Source: CAD feature listing. Evaluate the final solid. Frame: model axes, mm. Face numbers are marked on the shaded views. Give positions to 0.01 mm unless a question says otherwise; leave off trailing zeros. Write each loop counter-clockwise with the first axis right and the second up, starting at its lowest first coordinate (ties: lowest second). Pieces come first, ordered by that corner, then holes. Notation, with made-up numbers: M 41.5,-37 L 94.5,-37 A30 cw 94.5,-9 Z; hole C 30,-15.5 d5. An arc over 180 degrees is marked long. Return JSON: item names as keys, results as strings.
```python
from build123d import *

# Parameters (mm, degrees)
F0_W     = 88.9
F0_H     = 101.6
F1_DEPTH = 6.35
F2_R     = 5.08
F3_T     = -2.54
F4_W     = 83.82
F4_H     = 2.54
F5_DEPTH = 10.16
F7_DEPTH = 6.35
F8_R     = 5.08


with BuildPart() as f1:
    # F0 (on Front) → F1 (new body, symmetric)
    with BuildSketch(Plane.XZ):
        with Locations((0, 50.8)):
            Rectangle(F0_W, F0_H)
    extrude(amount=F1_DEPTH, both=True)

    # F2
    f2_edges = [f1.edges().sort_by_distance(p)[0] for p in [
        (-44.45, 0, 0),
        (44.45, 0, 0),
    ]]
    fillet(f2_edges, radius=F2_R)

    # F3
    f3_openings = [f1.faces().sort_by_distance(p)[0] for p in [
        (0, -6.35, 50.860979),
    ]]
    offset(amount=F3_T, openings=f3_openings)

    # F4 (on face) → F5 (cut, through all)
    with BuildSketch(Plane.XZ.offset(6.35)):
        with Locations((0, 100.33)):
            Rectangle(F4_W, F4_H)
    extrude(amount=-F5_DEPTH, mode=Mode.SUBTRACT)

    # F6 (on face) → F7 (join)
    with BuildSketch(Plane.XZ.offset(-3.81)):
        with BuildLine():
            Line((38.735, 5.715), (-38.735, 5.715))
            Line((-38.735, 5.715), (-38.735, 101.6))
            Line((-38.735, 101.6), (-41.91, 101.6))
            Line((-41.91, 101.6), (-41.91, 5.08))
            ThreePointArc((-41.91, 5.08), (-41.1660512242, 3.2839487758), (-39.37, 2.54))
            Line((-39.37, 2.54), (39.37, 2.54))
            ThreePointArc((39.37, 2.54), (41.1660512242, 3.2839487758), (41.91, 5.08))
            Line((41.91, 5.08), (41.91, 101.6))
            Line((41.91, 101.6), (38.735, 101.6))
            Line((38.735, 101.6), (38.735, 5.715))
        make_face()
    extrude(amount=F7_DEPTH)

    # F8
    f8_edges = [f1.edges().sort_by_distance(p)[0] for p in [
        (-38.735, 0.635, 5.715),
        (38.735, 0.635, 5.715),
    ]]
    fillet(f8_edges, radius=F8_R)


solid = f1.part
```
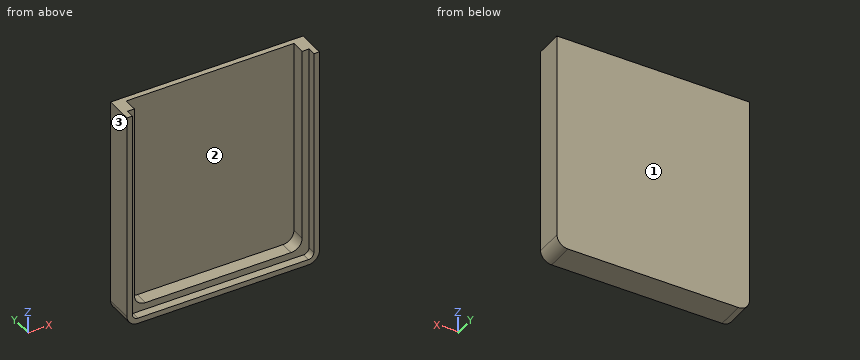
1) Cut plane C-C, the plane z = 81.5. Return the cut outline in (x, y) (3 decimals), then the cut area to 3 significant figures.
Numbers:
{"outline": "M -44.45,-6.35 L -41.91,-6.35 L -41.91,-2.54 L -38.735,-2.54 L -38.735,3.81 L 38.735,3.81 L 38.735,-2.54 L 41.91,-2.54 L 41.91,-6.35 L 44.45,-6.35 L 44.45,6.35 L -44.45,6.35 Z", "area": "318 mm²"}
2) Contact query for flat-ended pins moving along their axis: pin 1 Ø3 at (x, z) = (6.5, 39.5) entering from -Y; pin 2 Ø3 at (x, y) = (-4, 1) entering from +Z (3 decimals); pin 3 Ø4 at (x, y) = (11, -5) entering from +Z. Output: stop coordinate, or through.
Numbers:
{"pin 1": "stops at y = 3.81", "pin 2": "stops at z = 5.715", "pin 3": "stops at z = 2.54"}
3) Cut plane A-A, the plane y = 2.25. Return the cut outline in (x, z) (3 decimals).
Numbers:
{"outline": "M -44.45,5.08 A5.08 ccw -39.37,0 L 39.37,0 A5.08 ccw 44.45,5.08 L 44.45,101.6 L 38.735,101.6 L 38.735,10.795 A5.08 cw 33.655,5.715 L -33.655,5.715 A5.08 cw -38.735,10.795 L -38.735,101.6 L -44.45,101.6 Z"}
4) Line query: line 1 (X direction, y = 1.5, z = 35) (3 decimals); line 2 (X direction, y = -4, z = 36); line 3 (Z direction, x = 30, y = -2.75). Output: solid intervals per line, ascending. Write a range as [from, to].
Numbers:
{"line 1": "x = [-44.45, -38.735], [38.735, 44.45]", "line 2": "x = [-44.45, -41.91], [41.91, 44.45]", "line 3": "z = [0, 2.54]"}
5) Cut plane D-D, the plane x = 36. Return the cut outline in (y, z), then the cut area to 3 significant figures.
Numbers:
{"outline": "M -6.35,0 L 6.35,0 L 6.35,101.6 L 3.81,101.6 L 3.81,6.29 L -2.54,6.29 L -2.54,2.54 L -6.35,2.54 Z", "area": "308 mm²"}
6) Draft query along X for the marked faces 1, 2 and 3. Return one class per face: released by +X, released by -X, zero draft, split by the parting line, or undercut.
Numbers:
{"face 1": "zero draft", "face 2": "undercut", "face 3": "released by -X"}
7) Cut plane B-B, the plane x = -8. Return the cut outline in (y, z) (3 decimals).
Numbers:
{"outline": "M -6.35,0 L 6.35,0 L 6.35,101.6 L 3.81,101.6 L 3.81,5.715 L -2.54,5.715 L -2.54,2.54 L -6.35,2.54 Z"}
